from build123d import *

# Parameters (mm, degrees)
SKETCH3_R             = 4
BOSS_EXTRUDE1_DEPTH   = 290
M4_TAPPED_HOLE1_D     = 3.3
M4_TAPPED_HOLE1_DEPTH = 2.4
M4_TAPPED_HOLE1_TIP   = 0.991420021
M4_TAPPED_HOLE2_D     = 3.3
M4_TAPPED_HOLE2_DEPTH = 2.4
M4_TAPPED_HOLE2_TIP   = 0.991420021


with BuildPart() as part:
    # Sketch3 → Boss-Extrude1 (new body)
    with BuildSketch(Plane(origin=(0, 0, 0), x_dir=(1, 0, 0), z_dir=(0, 1, 0))):
        Circle(SKETCH3_R)
    extrude(amount=BOSS_EXTRUDE1_DEPTH)

    # M4 Tapped Hole1
    with Locations(Plane(origin=(0, 290, 0), x_dir=(1, 0, 0), z_dir=(0, 1, 0))):
        with Locations((0, 0)):
            Hole(M4_TAPPED_HOLE1_D / 2, depth=M4_TAPPED_HOLE1_DEPTH)
            with Locations((0, 0, -(M4_TAPPED_HOLE1_DEPTH + M4_TAPPED_HOLE1_TIP / 2))):  # 118° drill point
                Cone(0, M4_TAPPED_HOLE1_D / 2, M4_TAPPED_HOLE1_TIP, mode=Mode.SUBTRACT)

    # M4 Tapped Hole2
    with Locations(Plane(origin=(0, 0, 0), x_dir=(-1, 0, 0), z_dir=(0, -1, 0))):
        with Locations((0, 0)):
            Hole(M4_TAPPED_HOLE2_D / 2, depth=M4_TAPPED_HOLE2_DEPTH)
            with Locations((0, 0, -(M4_TAPPED_HOLE2_DEPTH + M4_TAPPED_HOLE2_TIP / 2))):  # 118° drill point
                Cone(0, M4_TAPPED_HOLE2_D / 2, M4_TAPPED_HOLE2_TIP, mode=Mode.SUBTRACT)


solid = part.part
Input: part model. Units: mm. Frame: model coordinates. Coordinates: 2 decimals unless noted, no trailing zeros. Loops run counter-clockwise (first coordinate to the right, second up) from the corner with the lowest first, then second, coordinate; pieces in that order, holes last.
(1) Pull-direction query (Z, two-part tool) for faces 1 (the face through (2, 290, 0)), 2 (the face through (-0.867, 142.97, 3.905)); classes: released by +Z, released by -Z, zero draft, split by the parting line, or undercut.
(2) Material intervals for probe 1 along Z at (x, y) = (0, 1.55); probe 2 along X at (y, z) = (120, 0.25); probe 3 along Y at (x, z) = (0.75, 0.25), sorted ascending.
(3) First-contact query: pin 1 Ø2.5 at (x, z) = (0, 0) entering from -Y. Flat tip, straight axial feed; report the tip coordinate or a pass-through.
(4) Section A-A on y = 160. Return the cut outline in (x, z), then the cut area to 3 significant figures.
Data:
1. face 1: zero draft
1. face 2: split by the parting line
2. probe 1: z = -4 to -1.65, 1.65 to 4
2. probe 2: x = -3.99 to 3.99
2. probe 3: y = 2.92 to 287.08
3. pin 1: stops at y = 2.64
4. outline: circle Ø8 at (0, 0)
4. area: 50.3 mm2
